Work out the finished part from the listing and answer in its coordinate system (mm). A direction names the side the tool comes from. Give positions to 0.01 mm unless a question says otherwise; leave off trailing zeros. Loops run counter-clockwise (first coordinate to the right, second up) from the corner with the lowest first, then second, coordinate; pieces in that order, holes last. Notation, with made-up numbers: M 16,80 L 23,80 A18 ccw 23,104 Z; hole C 58.25,85 d3. An arc over 180 degrees is marked long. Answer in a Markdown table with one row per item. Add a question column.
from build123d import *

# Parameters (mm, degrees)
CROQUIS1_R              = 1.25
SALIENTE_EXTRUIR1_DEPTH = 15
CROQUIS4_R              = 22.5
SALIENTE_EXTRUIR2_DEPTH = 15
CROQUIS5_R              = 11
CORTAR_EXTRUIR1_DEPTH   = 5
CROQUIS6_W              = 40
CROQUIS6_H              = 42
CORTAR_EXTRUIR2_DEPTH   = 5


with BuildPart() as part:
    # Croquis1 → Saliente-Extruir1 (new body)
    with BuildSketch(Plane.XY):
        with BuildLine():
            Line((0, -50), (215, -40))
            ThreePointArc((215, -40), (255, 0), (215, 40))
            Line((215, 40), (0, 50))
            ThreePointArc((0, 50), (-50, 0), (0, -50))
        make_face()
        Circle(CROQUIS1_R, mode=Mode.SUBTRACT)
        with Locations((215, 0)):
            Circle(CROQUIS1_R, mode=Mode.SUBTRACT)
    extrude(amount=SALIENTE_EXTRUIR1_DEPTH)

    # Croquis4 → Saliente-Extruir2 (add)
    with BuildSketch(Plane.XY.offset(15)):
        Circle(CROQUIS4_R)
    extrude(amount=SALIENTE_EXTRUIR2_DEPTH)

    # Croquis5 → Cortar-Extruir1 (cut)
    with BuildSketch(Plane(origin=(0, 0, 0), x_dir=(-1, 0, 0), z_dir=(0, 0, -1))):
        Circle(CROQUIS5_R)
    extrude(amount=-CORTAR_EXTRUIR1_DEPTH, mode=Mode.SUBTRACT)

    # Croquis6 → Cortar-Extruir2 (cut)
    with BuildSketch(Plane.XY.offset(15)):
        with Locations((215, 0)):
            Rectangle(CROQUIS6_W, CROQUIS6_H)
    extrude(amount=-CORTAR_EXTRUIR2_DEPTH, mode=Mode.SUBTRACT)


solid = part.part
(1) Which of the six approach directions +Z, -Z, +X, -X, +Y, -Y give full straight-line access (tool end or side, diameter ignored) to faces 1 (the face through (254.99, -0.88, 7.4)), 2 (the face through (215, -21, 13)), 3 (the face through (2.38, -10.74, 2.46))?
(2) Section A-A, the plane x = 119.5 is taken. Determine the outline of the cut face in (y, z), and give its area (3 significant figures).
(3) Each of these flat-tipped pins is pushed along its axis until it touches: P1, Ø1, axis at x = 174, z = 9, coming from the -Y side; P2, Ø8, axis at y = 39, z = 16, coming from the -X side; P3, Ø1, axis at x = 97.5, z = 6, coming from the -Y side; P4, Ø2, axis at x = 215, y = 0, coming from the +Z side. Where does it stop, or does it pass through?
(4) Section B-B, the plane y = -44 is taken. Determine the outline of the cut face in (x, z), and give its area (3 significant figures).
(5) The mould has two halves that part along Y. Classify faces 4 (the face through (109, 44.93, 7.4)), 5 (the face through (210, 0, 10)), 6 (the face through (100, 1, 15)): pulls with the +Y half, pulls with the -Y half, needs draft (parallel to the pull), parting line crosses it, or undercut.
(6) Consider line 1 along X through (y, z) = (0, 6); line 2 along Y through (x, z) = (0, 12.5); line 3 along Y through (x, z) = (0, 3.8). Determine where each line is inside the solid, lowest interval first. Write a range as from..to.
Numbers:
| question | item | result |
|---|---|---|
| 1 | face 1 | +Z, -Z, +X |
| 1 | face 2 | +Z |
| 1 | face 3 | -Z |
| 2 | outline | M -44.44,0 L 44.44,0 L 44.44,15 L -44.44,15 Z |
| 2 | area | 1,330 mm² |
| 3 | P1 | stops at y = -41.93 |
| 3 | P2 | stops at x = -35.58 |
| 3 | P3 | stops at y = -45.49 |
| 3 | P4 | passes through |
| 4 | outline | M -23.75,0 L 129,0 L 129,15 L -23.75,15 Z |
| 4 | area | 2,290 mm² |
| 5 | face 4 | pulls with the +Y half |
| 5 | face 5 | undercut |
| 5 | face 6 | needs draft |
| 6 | line 1 | x = -50..-1.25, 1.25..213.75, 216.25..255 |
| 6 | line 2 | y = -50..-1.25, 1.25..50 |
| 6 | line 3 | y = -50..-11, 11..50 |
